The figure shows three views and two pictorial views of one solid part (mm, origin at its lowest corner). Answer the questions. Coordinates: 2 decimals unless noted, no trailing zeros. Order: outer loops, then holes, each group sorted by start corner. A loop starts at its lowest first (then second) coordinate and runs counter-clockwise, first axis right, second up. Notation, with made-up numbers: (77, 55) -> (109, 55) arc R26 cw to (109, 90) -> close; hole circle Ø5 at (49, -31). An arc over 180 degrees is marked (long way). Write item = value, one per line.
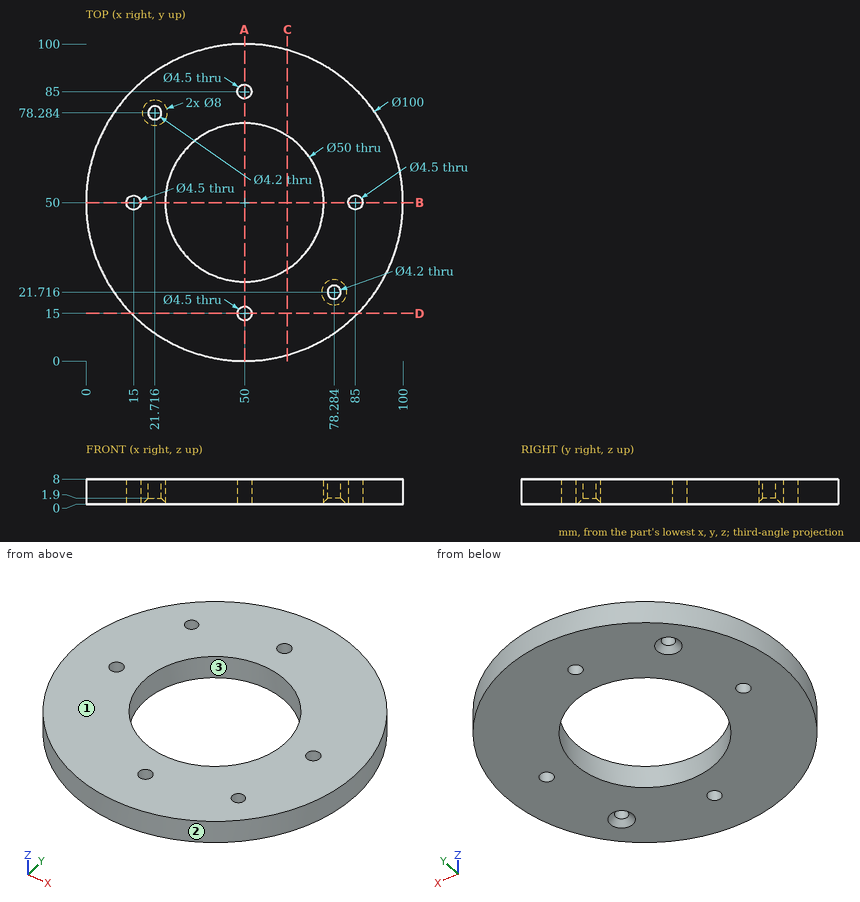
Q1. Each of these flat-tipped pins is pushed along its axis until it touches: pin 1 Ø3 at (x, z) = (44.5, 5.5) entering from -Y; pin 2 Ø2 at (x, z) = (18.5, 4.5) entering from +Y; pin 3 Ø3 at (x, z) = (63.5, 5.5) entering from +Y. Where does it stop, or does it pass through?
The answers:
pin_1 = 0.16
pin_2 = 89.62
pin_3 = 98.54
Q2. Section D-D, the plane y = 15 is taken. Give the vertices of the cut face in (x, z), plus the area to 3 significant figures.
The answers:
outline = (14.29, 0) -> (47.75, 0) -> (47.75, 8) -> (14.29, 8) -> close; (52.25, 0) -> (85.71, 0) -> (85.71, 8) -> (52.25, 8) -> close
area = 535 mm2
Q3. Section C-C, the plane x = 63.5 is taken. Give the vertices of the cut face in (y, z), plus the area to 3 significant figures.
The answers:
outline = (1.86, 0) -> (28.96, 0) -> (28.96, 8) -> (1.86, 8) -> close; (71.04, 0) -> (98.14, 0) -> (98.14, 8) -> (71.04, 8) -> close
area = 434 mm2
Q4. Section A-A, the plane x = 50 is taken. Give the vertices of the cut face in (y, z), plus the area to 3 significant figures.
The answers:
outline = (0, 0) -> (12.75, 0) -> (12.75, 8) -> (0, 8) -> close; (17.25, 0) -> (25, 0) -> (25, 8) -> (17.25, 8) -> close; (75, 0) -> (82.75, 0) -> (82.75, 8) -> (75, 8) -> close; (87.25, 0) -> (100, 0) -> (100, 8) -> (87.25, 8) -> close
area = 328 mm2
Q5. The mould has two halves that part along Y. Classify the marked faces 1, 2 and 3: released by +Y, released by -Y, zero draft, split by the parting line, or undercut.
The answers:
face_1 = zero draft
face_2 = split by the parting line
face_3 = undercut
Q6. Find the intervals of material crossed by line 1 along Y through (x, z) = (50, 5); line 2 along X through (y, z) = (39.5, 1.25) (1 decimal); line 3 along X through (y, z) = (57.5, 3) (1 decimal), in increasing order.
The answers:
line_1 = 0 to 12.75, 17.25 to 25, 75 to 82.75, 87.25 to 100
line_2 = 1.1 to 27.3, 72.7 to 98.9
line_3 = 0.6 to 26.2, 73.8 to 99.4
